The drawing under review shows one solid part. Ordinate dimensions are in mm from its lowest x, y, z. A direction names the side the tool comes from. Round coordinates to 2 decimals unless told otherwise and drop trailing zeros. Loops run counter-clockwise (first coordinate to the right, second up) from the corner with the lowest first, then second, coordinate; pieces in that order, holes last. Notation, with made-up numbers: (-23, -13.75) - (-7, -13.75) arc R24 ccw to (-7, 17.25) - close; hole circle Ø11 at (83.25, 1.5). An arc over 180 degrees is marked (long way). Answer as CSV lines item,"result".
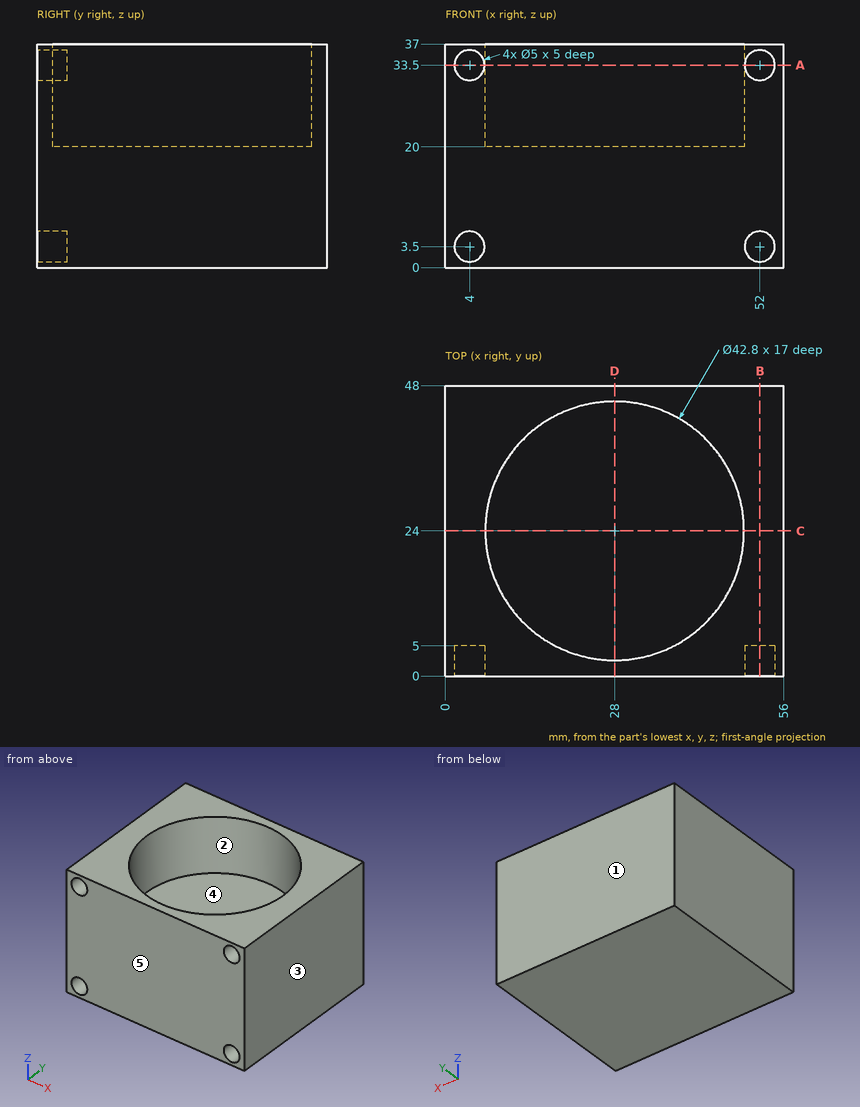
1. Wall thickness on probe 1 along X at (y, z) = (4, 3.5); probe 2 along X at (y, z) = (1, 33); probe 3 along Y at (x, z) = (28, 25.5): over which ranges is each line inside the solid? List them lowest first.
Numbers:
probe 1,"x = 0 to 1.5, 6.5 to 49.5, 54.5 to 56"
probe 2,"x = 0 to 1.55, 6.45 to 49.55, 54.45 to 56"
probe 3,"y = 0 to 2.6, 45.4 to 48"
2. Take a section at A-A (z = 33.5). State the section outline as (x, y) points, plus the area to 3 significant figures.
Numbers:
outline,"(0, 0) - (1.5, 0) - (1.5, 5) - (6.5, 5) - (6.5, 0) - (49.5, 0) - (49.5, 5) - (54.5, 5) - (54.5, 0) - (56, 0) - (56, 48) - (0, 48) - close; hole circle Ø42.8 at (28, 24)"
area,"1,200 mm²"
3. Tool access review of the marked faces 1 and 2: name each direction out of +Z, -Z, +X, -X, +Y, -Y from which nothing blocks a thin tool from reaching the whole face with its end or side.
Numbers:
face 1,"+Z, -Z, +X, -X, +Y"
face 2,"+Z"
4. Clearance check with flat-ended pins moving along their axes: pin 1 (5 mm diameter, centred on x = 39, y = 17.5, fed in from +Z); pin 2 (2.5 mm diameter, centred on x = 53, z = 33.5, fed in from -Y). State where each tip first meets the part, or that it passes through.
Numbers:
pin 1,"stops at z = 20"
pin 2,"stops at y = 5"
5. Take a section at D-D (x = 28). State the section outline as (y, z) points.
Numbers:
outline,"(0, 0) - (48, 0) - (48, 37) - (45.4, 37) - (45.4, 20) - (2.6, 20) - (2.6, 37) - (0, 37) - close"
6. Take a section at B-B (x = 52). State the section outline as (y, z) points.
Numbers:
outline,"(0, 0) - (48, 0) - (48, 37) - (0, 37) - (0, 36) - (5, 36) - (5, 31) - (0, 31) - (0, 6) - (5, 6) - (5, 1) - (0, 1) - close"
7. Take a section at C-C (y = 24). State the section outline as (x, z) points, plus the area to 3 significant figures.
Numbers:
outline,"(0, 0) - (56, 0) - (56, 37) - (49.4, 37) - (49.4, 20) - (6.6, 20) - (6.6, 37) - (0, 37) - close"
area,"1,340 mm²"
8. Draft analysis for pull direction X (two halves, no side actions). For the marked faces 3, 4 and 5, state which applies: +X half, -X half, draft (parallel to the pull), parting line (faces both ways), or undercut.
Numbers:
face 3,"+X half"
face 4,"undercut"
face 5,"draft"
